Check sheet for the drawn part. Datum: minimum x, y, z corner. Units: mm. A direction names the side the tool comes from. Round coordinates to 2 decimals unless told otherwise and drop trailing zeros. Write each loop counter-clockwise with the first axis right and the second up, starting at its lowest first coordinate (ties: lowest second). Pieces come first, ordered by that corner, then holes. Notation, with made-up numbers: (65, -10.5) - (108, -10.5) arc R28 cw to (108, 13.5) - close; hole circle Ø10 at (-23.5, -30). An arc over 180 degrees is marked (long way). Answer as a JSON object with one key per item and string values. Group by question number.
1) Set-up check for the marked faces 1 and 2: record each of +Z, -Z, +X, -X, +Y, -Y from which the full face is reachable in a straight line by a thin tool's end or side.
2) Thickness scan on line 1 (X direction, y = 67, z = 23.5); line 2 (Z direction, x = 149, y = 38.1); line 3 (Z direction, x = 90, y = 45). Record the ranges inside material, lowest first.
3) Section check A-A (z = 50.8). Enter the section's corners in (x, y), then the cut area to 3 significant figures.
4) Go/stop test with a flat-tipped pin: pin 1 Ø10 at (x, y) = (29, 67.5) entering from +Z. Record where the tip stops, or that it passes through.
5) Section check C-C (y = 66). Enter the section's corners in (x, z), then the cut area to 3 significant figures.
6) Section check D-D (x = 127.5). Enter the section's corners in (y, z), then the cut area to 3 significant figures.
7) Section check B-B (y = 38). Enter the section's corners in (x, z), then the cut area to 3 significant figures.
8) Mould release check, pull along X, two halves, no side actions. Record for the marked faces 3, 4 and 5: +X half, -X half, draft (parallel to the pull), parting line (faces both ways), or undercut.
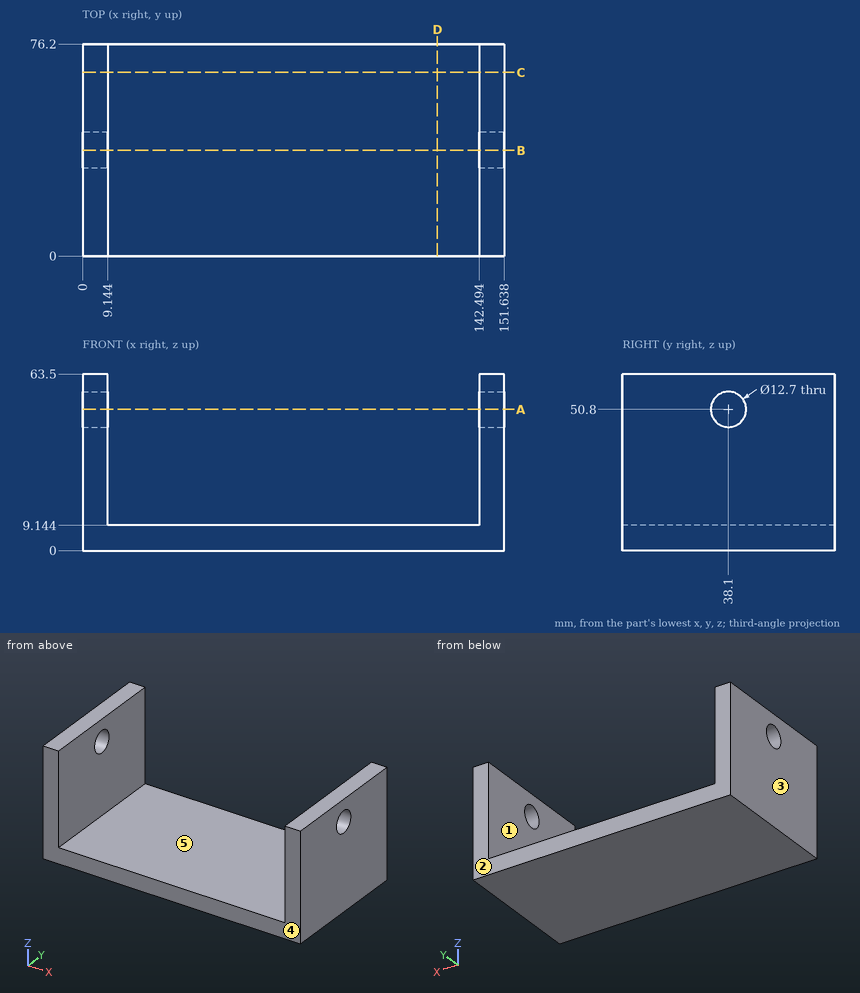
Returned:
{
 "1": {"face 1": "+Z, +Y, -Y", "face 2": "+Z, -Z, +X, -X, +Y"},
 "2": {"line 1": "0 to 9.14, 142.49 to 151.64", "line 2": "0 to 44.45, 57.15 to 63.5", "line 3": "0 to 9.14"},
 "3": {"outline": "(0, 0) - (9.14, 0) - (9.14, 31.75) - (0, 31.75) - close; (0, 44.45) - (9.14, 44.45) - (9.14, 76.2) - (0, 76.2) - close; (142.49, 0) - (151.64, 0) - (151.64, 31.75) - (142.49, 31.75) - close; (142.49, 44.45) - (151.64, 44.45) - (151.64, 76.2) - (142.49, 76.2) - close", "area": "1,160 mm2"},
 "4": {"pin 1": "z = 9.14"},
 "5": {"outline": "(0, 0) - (151.64, 0) - (151.64, 63.5) - (142.49, 63.5) - (142.49, 9.14) - (9.14, 9.14) - (9.14, 63.5) - (0, 63.5) - close", "area": "2,380 mm2"},
 "6": {"outline": "(0, 0) - (76.2, 0) - (76.2, 9.14) - (0, 9.14) - close", "area": "697 mm2"},
 "7": {"outline": "(0, 0) - (151.64, 0) - (151.64, 44.45) - (142.49, 44.45) - (142.49, 9.14) - (9.14, 9.14) - (9.14, 44.45) - (0, 44.45) - close; (0, 57.15) - (9.14, 57.15) - (9.14, 63.5) - (0, 63.5) - close; (142.49, 57.15) - (151.64, 57.15) - (151.64, 63.5) - (142.49, 63.5) - close", "area": "2,150 mm2"},
 "8": {"face 3": "-X half", "face 4": "draft", "face 5": "undercut"}
}
